Build history of the part. All positions in model axes, mm. Coordinates: 2 decimals unless noted, no trailing zeros. Write each loop counter-clockwise with the first axis right and the second up, starting at its lowest first coordinate (ties: lowest second). Pieces come first, ordered by that corner, then holes.
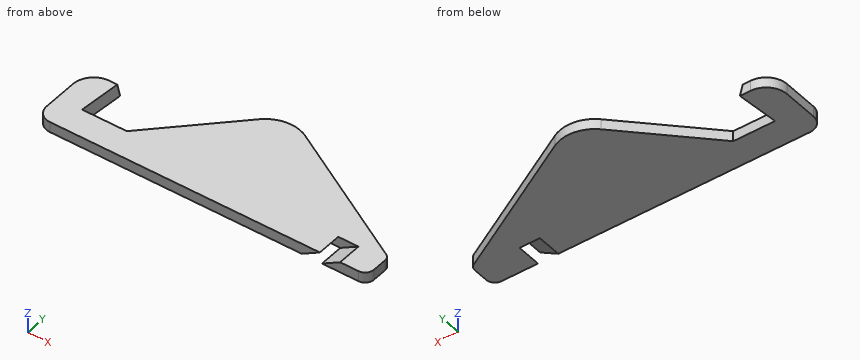
```python
from build123d import *

# Parameters (mm, degrees)
F1_DEPTH = 3
F5_SIZE2 = 0.803838
F5_SIZE  = 2.99999
F4_W     = 7
F4_H     = 2.9
F6_DEPTH = 12.5


# Not quite as in the source:
# - a fillet or chamfer is up to 0.001 mm smaller than in the source, because OpenCascade refuses the exact size


with BuildPart() as f1:
    # F0 (on Top) → F1 (new body)
    with BuildSketch(Plane.XY):
        with BuildLine():
            Line((4, 0), (92.5, 0))
            ThreePointArc((92.5, 0), (94.267766953, 0.732233047), (95, 2.5))
            Line((95, 2.5), (95, 6.8303050312))
            ThreePointArc((95, 6.8303050312), (94.7264189756, 7.8399968261), (93.9805224793, 8.5734561054))
            Line((93.9805224793, 8.5734561054), (53.6105552952, 31.2815626464))
            ThreePointArc((53.6105552952, 31.2815626464), (47.3471346779, 32.4727846642), (41.636875087, 29.636875087))
            Line((41.636875087, 29.636875087), (20, 8))
            Line((20, 8), (8, 8))
            Line((8, 8), (9.0498639623, 20))
            Line((9.0498639623, 20), (6, 20))
            ThreePointArc((6, 20), (1.7573593129, 18.2426406871), (0, 14))
            Line((0, 14), (0, 4))
            ThreePointArc((0, 4), (1.1715728753, 1.1715728753), (4, 0))
        make_face()
    extrude(amount=F1_DEPTH)

    # F5 (size 3 and 0.8038475773 in the source; OpenCascade refuses exactly that, so slightly less here)
    f5_edges = [f1.edges().sort_by_distance(p)[0] for p in [
        (8.524932, 14, 3),
    ]]
    f5_side = f1.faces().sort_by_distance((8.524932, 14, 1.5))[0]
    chamfer(f5_edges, length=F5_SIZE, length2=F5_SIZE2, reference=f5_side)

    # F4 (on line) → F6 (cut, symmetric)
    with BuildSketch(Plane(origin=(61.5, 0, 35.5070415552), x_dir=(0, 1, 0), z_dir=(0.8660254038, 0, 0.5))):
        with Locations((3.5, -39.55)):
            Rectangle(F4_W, F4_H)
    extrude(amount=F6_DEPTH, both=True, mode=Mode.SUBTRACT)


solid = f1.part
```
1. Saw through at C-C on x = 26. List the corners of the cut face in (y, z).
Computed values:
outline: (0, 0) - (14, 0) - (14, 3) - (0, 3) - close
2. Probe line 1 along X through (y, z) = (3, 2.3); line 2 along X through (y, z) = (11.5, 1); line 3 along Y through (x, z) = (64.5, 1.55). List the from-to ranges inside material, lowest first.
Computed values:
line 1: x = 0.13 to 80.18, 85.98 to 95
line 2: x = 0 to 8.04, 23.5 to 88.78
line 3: y = 0 to 25.16
3. Saw through at D-D on y = 21.5. List the corners of the cut face in (x, z).
Computed values:
outline: (33.5, 0) - (71, 0) - (71, 3) - (33.5, 3) - close
4. Flat gauge pin, fed straight in: pin 1 (1.5 mm diameter, centred on x = 11.5, z = 2.5, fed in from +Y). Where does the tip first touch, or does it go through?
Computed values:
pin 1: stops at y = 8
5. Saw through at B-B on z = 1.4. List the corners of the cut face in (x, y), plus the area to 3 significant figures.
Computed values:
outline: (0, 4) arc R4 ccw to (4, 0) - (78.62, 0) - (78.62, 7) - (84.42, 7) - (84.42, 0) - (92.5, 0) arc R2.5 ccw to (95, 2.5) - (95, 6.83) arc R2 ccw to (93.98, 8.57) - (53.61, 31.28) arc R10 ccw to (41.64, 29.64) - (20, 8) - (7.62, 8) - (8.67, 20) - (6, 20) arc R6 ccw to (0, 14) - close
area: 1,810 mm2
